The model under review builds one solid part; all positions refer to its coordinate system, in mm. A direction names the side the tool comes from. Round coordinates to 2 decimals unless told otherwise and drop trailing zeros. Order: outer loops, then holes, each group sorted by start corner. A loop starts at its lowest first (then second) coordinate and runs counter-clockwise, first axis right, second up.
```python
from build123d import *

# Parameters (mm, degrees)
SKETCH1_R               = 2.24506403
BOSS_EXTRUDE1_DEPTH     = 3
FILLET1_R               = 2.54
SKETCH2_R               = 2.2479
TORQUE_PREVENTION_DEPTH = 136.15202741


with BuildPart() as part:
    # Sketch1 → Boss-Extrude1 (new body)
    with BuildSketch(Plane(origin=(0, 0, 0), x_dir=(0, 0, -1), z_dir=(1, 0, 0))):
        with BuildLine():
            Line((0, -6.35), (66.675, -6.35))
            Line((66.675, -6.35), (66.675, -56.962915387))
            Line((66.675, -56.962915387), (115.296830482, -58.417161651))
            ThreePointArc((115.296830482, -58.417161651), (121.833831472, -52.259839338), (115.676509159, -45.722838349))
            Line((115.676509159, -45.722838349), (79.375, -44.637084613))
            Line((79.375, -44.637084613), (79.375, 6.35))
            Line((79.375, 6.35), (0, 6.35))
            ThreePointArc((0, 6.35), (-6.35, 0), (0, -6.35))
        make_face()
        with Locations((115.486669821, -52.07)):
            Circle(SKETCH1_R, mode=Mode.SUBTRACT)
        Polygon((0, 2.24506403), (2.24506403, 0), (0, -2.24506403), (-2.24506403, 0), align=None, mode=Mode.SUBTRACT)
    extrude(amount=BOSS_EXTRUDE1_DEPTH)

    # Fillet1
    fillet1_edges = [part.edges().sort_by_distance(p)[0] for p in [
        (1.5, 6.35, -79.375),
        (1.5, -44.637084613, -79.375),
        (1.5, -56.962915387, -66.675),
        (1.5, -6.35, -66.675),
    ]]
    fillet(fillet1_edges, radius=FILLET1_R)

    # Sketch2 → Torque prevention (cut, through all)
    with BuildSketch(Plane(origin=(3, 0, 0), x_dir=(0, 0, -1), z_dir=(1, 0, 0))):
        with Locations((73.742299151, -50.103834019)):
            Circle(SKETCH2_R)
        with Locations((61.042299151, 0)):
            Circle(SKETCH2_R)
    extrude(amount=-TORQUE_PREVENTION_DEPTH, mode=Mode.SUBTRACT)


solid = part.part
```
(1) Consider section A-A (x = 1.75). State how many separate pieces and enclosed holes the cut face has, and give its area (3 significant figures).
Data:
separate pieces: 1
enclosed holes: 4
area: 2,180 mm2
(2) Insertion check: pin 1 (6 mm diameter, centred on y = -50.1, z = -73.74, fed in from -X); pin 2 (1.5 mm diameter, centred on x = 2, y = -9, fed in from -Z) (3 decimals). Each pin has a flat end and moves straight along its axis. Give the tip position at first contact, or say it passes through.
Data:
pin 1: stops at x = 0
pin 2: stops at z = -79.375
(3) To check wall thickness, follow probe 1 along Z at (x, y) = (2.15, -50.5) (3 decimals); probe 2 along Z at (x, y) = (2.75, -51) (3 decimals); probe 3 along Y at (x, z) = (0.3, -35). State the ranges of each line that lie inside material, in increasing order.
Data:
probe 1: z = -121.64 to -117.091, -113.882 to -75.955, -71.53 to -66.675
probe 2: z = -121.746 to -117.46, -113.513 to -75.804, -71.681 to -66.675
probe 3: y = -6.35 to 6.35
(4) For faces 4 (the flat face through (1.479, 1.138, -1.107)), 5 (the flat face through (1, -20, -79.375)), 6 (the flat face through (1, -31, -66.675)), list the 3-axis set-ups (+Z, -Z, +X, -X, +Y, -Y) from which the entire face can be reached by the end or side of a thin tool; tool diameter is ignored.
Data:
face 4: +X, -X
face 5: -Z, +X, -X, +Y
face 6: +Z, +X, -X, -Y
(5) Draft analysis for pull direction Y (two halves, no side actions). For faces 1 (the flat face through (1.479, -1.138, 1.107)), 2 (the flat face through (0, -21, -67)), 3 (the cylindrical face through (1.48, 0.14, 6.35)), state which applies: pulls with the +Y half, pulls with the -Y half, needs draft (parallel to the pull), parting line crosses it, or undercut.
Data:
face 1: undercut
face 2: needs draft
face 3: parting line crosses it
(6) Consider section B-B (z = -29.5). Write out the cut boundary in (x, y), and give its area (3 significant figures).
Data:
outline: (0, -6.35) - (3, -6.35) - (3, 6.35) - (0, 6.35) - close
area: 38.1 mm2
(7) Consider section C-C (y = -33). Write out the cut boundary in (x, z) (3 decimals).
Data:
outline: (0, -79.375) - (3, -79.375) - (3, -66.675) - (0, -66.675) - close
